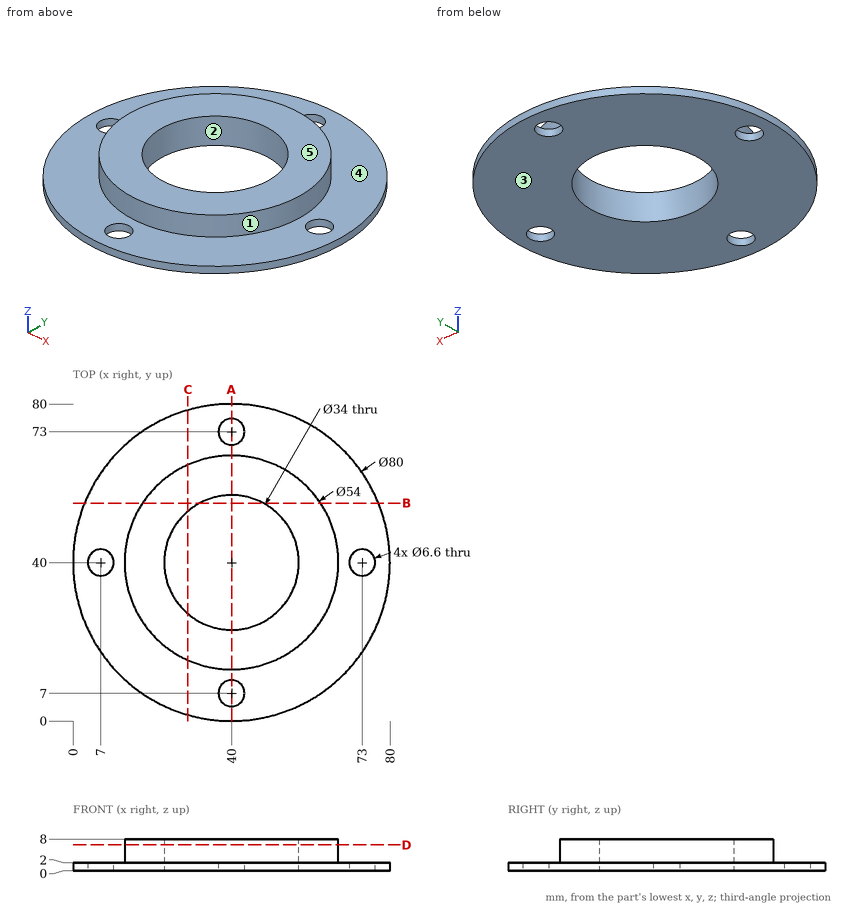
Drawing for the job (mm, zero at the part's lowest x, y, z). A direction names the side the tool comes from. Give positions to 0.01 mm unless a question says otherwise; leave off trailing zeros. Write each loop counter-clockwise with the first axis right and the second up, starting at its lowest first coordinate (ties: lowest second). Pieces come first, ordered by that corner, then holes. Notation, with made-up numbers: M 6,-38.5 L 49,-38.5 A15 cw 49,-28.5 Z; hole C 85,31 d9. An arc over 180 degrees is marked long. Return JSON: item names as keys, results as strings. Group by question number.
(1) Drill centre lines: L1, parallel to Y at x = 40, z = 3; L2, parallel to Z at x = 8.5, y = 61.5; L3, parallel to Y at x = 27, z = 4. Where is each one in solid material? Low to high. Write a range as [from, to].
(2) Band-saw the part on C-C (x = 29). Give the cut face in (y, z).
(3) Flat gauge pins, fed straight in: pin 1 Ø24 at (x, y) = (30.5, 27.5) entering from +Z; pin 2 Ø3 at (x, z) = (40, 3) entering from -Y; pin 3 Ø3 at (y, z) = (53.5, 4.5) entering from +X; pin 4 Ø7.5 at (x, y) = (40, 7) entering from +Z. Where does each tip first touch, or does it go through?
(4) Band-saw the part on B-B (y = 55). Give the cut face in (x, z), and give its area (3 significant figures).
(5) Mould opens along X. For the marked faces 1, 2 and 3 say: pulls with the +X half, pulls with the -X half, needs draft (parallel to the pull), parting line crosses it, or undercut.
(6) Band-saw the part on D-D (z = 6.5). Give the cut face in (x, y).
(7) Band-saw the part on A-A (x = 40). Give the cut face in (y, z).
(8) 3-axis set-ups, long thin cutter, end or side, ignore diameter. For the marked faces 4 and 5: which of +Z, -Z, +X, -X, +Y, -Y reach the whole face in a straight line?
Entries:
{
 "1": {"L1": "y = [13, 23], [57, 67]", "L2": "z = [0, 2]", "L3": "y = [16.34, 29.05], [50.95, 63.66]"},
 "2": {"outline": "M 1.54,0 L 27.04,0 L 27.04,8 L 15.34,8 L 15.34,2 L 1.54,2 Z; M 52.96,0 L 78.46,0 L 78.46,2 L 64.66,2 L 64.66,8 L 52.96,8 Z"},
 "3": {"pin 1": "stops at z = 8", "pin 2": "stops at y = 0", "pin 3": "stops at x = 64.19", "pin 4": "stops at z = 2"},
 "4": {"outline": "M 2.92,0 L 32,0 L 32,8 L 17.55,8 L 17.55,2 L 2.92,2 Z; M 48,0 L 77.08,0 L 77.08,2 L 62.45,2 L 62.45,8 L 48,8 Z", "area": "290 mm^2"},
 "5": {"face 1": "parting line crosses it", "face 2": "undercut", "face 3": "needs draft"},
 "6": {"outline": "C 40,40 d54; hole C 40,40 d34"},
 "7": {"outline": "M 0,0 L 3.7,0 L 3.7,2 L 0,2 Z; M 10.3,0 L 23,0 L 23,8 L 13,8 L 13,2 L 10.3,2 Z; M 57,0 L 69.7,0 L 69.7,2 L 67,2 L 67,8 L 57,8 Z; M 76.3,0 L 80,0 L 80,2 L 76.3,2 Z"},
 "8": {"face 4": "+Z", "face 5": "+Z, +X, -X, +Y, -Y"}
}
